```python
from build123d import *

# Parameters (mm, degrees)
F1_DEPTH = 0.635


# Not quite as in the source:
# - a feature names something its author has since deleted; it is built from what else it names


with BuildPart() as f1:
    # F0 (on Top) → F1 (new body)
    with BuildSketch(Plane.XY):
        with BuildLine():
            ThreePointArc((107.95, 0), (107.0200640303, 2.2450640303), (104.775, 3.175))
            Line((104.775, 3.175), (-69.215, 3.175))
            Line((-69.215, 3.175), (-74.295, 3.175))
            Line((-74.295, 3.175), (-74.295, -3.175))
            Line((-74.295, -3.175), (-69.215, -3.175))
            Line((-69.215, -3.175), (104.775, -3.175))
            ThreePointArc((104.775, -3.175), (107.0200640303, -2.2450640303), (107.95, 0))
        make_face()
        with BuildLine():
            Line((-74.295, -3.175), (-74.295, 3.175))
            Line((-74.295, 3.175), (-79.375, 3.175))
            Line((-79.375, 3.175), (-104.775, 3.175))
            ThreePointArc((-104.775, 3.175), (-107.0200640303, 2.2450640303), (-107.95, 0))
            ThreePointArc((-107.95, 0), (-107.0200640303, -2.2450640303), (-104.775, -3.175))
            Line((-104.775, -3.175), (-79.375, -3.175))
            Line((-79.375, -3.175), (-74.295, -3.175))
        make_face()
        with BuildLine():
            Line((-74.295, 9.525), (-69.215, 9.525))
            Line((-69.215, 9.525), (104.775, 9.525))
            ThreePointArc((104.775, 9.525), (107.0200640303, 10.4549359697), (107.95, 12.7))
            ThreePointArc((107.95, 12.7), (107.0200640302, 14.9450640302), (104.775, 15.875))
            Line((104.775, 15.875), (-74.295, 15.875))
            Line((-74.295, 15.875), (-74.295, 9.525))
        make_face()
        with BuildLine():
            Line((-79.375, 9.525), (-74.295, 9.525))
            Line((-74.295, 9.525), (-74.295, 15.875))
            Line((-74.295, 15.875), (-104.775, 15.875))
            ThreePointArc((-104.775, 15.875), (-107.0200640302, 14.9450640302), (-107.95, 12.7))
            ThreePointArc((-107.95, 12.7), (-107.0200640303, 10.4549359697), (-104.775, 9.525))
            Line((-104.775, 9.525), (-79.375, 9.525))
        make_face()
        with BuildLine():
            Line((-69.2150000001, -9.5250000001), (-74.295, -9.5250000001))
            Line((-74.295, -9.5250000001), (-74.295, -15.875))
            Line((-74.295, -15.875), (104.775, -15.875))
            ThreePointArc((104.775, -15.875), (107.0200640302, -14.9450640302), (107.95, -12.7))
            ThreePointArc((107.95, -12.7), (107.0200640303, -10.4549359697), (104.775, -9.525))
            Line((104.775, -9.5250000001), (-69.2150000001, -9.5250000001))
        make_face()
        with BuildLine():
            Line((-74.295, -15.875), (-74.295, -9.5250000001))
            Line((-74.295, -9.5250000001), (-79.375, -9.5250000001))
            Line((-79.375, -9.5250000001), (-104.775, -9.5250000001))
            ThreePointArc((-104.775, -9.525), (-107.0200640303, -10.4549359697), (-107.95, -12.7))
            ThreePointArc((-107.95, -12.7), (-107.0200640302, -14.9450640302), (-104.775, -15.875))
            Line((-104.775, -15.875), (-74.295, -15.875))
        make_face()
        with BuildLine():
            Line((-79.375, 3.175), (-74.295, 3.175))
            Line((-74.295, 3.175), (-74.295, 9.525))
            Line((-74.295, 9.525), (-79.375, 9.525))
            ThreePointArc((-79.375, 9.525), (-77.98351653, 6.35), (-79.375, 3.175))
        make_face()
        with BuildLine():
            Line((-74.295, 3.175), (-69.215, 3.175))
            ThreePointArc((-69.215, 3.175), (-70.6064834701, 6.35), (-69.215, 9.525))
            Line((-69.215, 9.525), (-74.295, 9.525))
            Line((-74.295, 9.525), (-74.295, 3.175))
        make_face()
        with BuildLine():
            Line((-74.295, -9.5250000001), (-74.295, -3.175))
            Line((-74.295, -3.175), (-79.375, -3.175))
            ThreePointArc((-79.375, -3.175), (-77.9835165299, -6.35), (-79.375, -9.525))
            Line((-79.375, -9.5250000001), (-74.295, -9.5250000001))
        make_face()
        with BuildLine():
            Line((-69.215, -3.175), (-74.295, -3.175))
            Line((-74.295, -3.175), (-74.295, -9.5250000001))
            Line((-74.295, -9.5250000001), (-69.2150000001, -9.5250000001))
            ThreePointArc((-69.2150000001, -9.525), (-70.6064834702, -6.35), (-69.215, -3.175))
        make_face()
    extrude(amount=F1_DEPTH)


solid = f1.part
```
The listing builds one solid part. Answer for the finished solid, in the listing's coordinates (mm). Give positions to 0.01 mm unless a question says otherwise; leave off trailing zeros. Order: outer loops, then holes, each group sorted by start corner. A loop starts at its lowest first (then second) coordinate and runs counter-clockwise, first axis right, second up. Notation, with made-up numbers: (-26.75, -12) -> (13.25, -12) arc R32 cw to (13.25, 17) -> close; hole circle Ø2 at (49.25, 8.5). An arc over 180 degrees is marked (long way). One line per item, written item: value.
1) Find section A-A, the plane x = -15. Determine the outline of the cut face in (y, z) (3 decimals), plus the area to 3 significant figures.
Reported:
outline: (-15.875, 0) -> (-9.525, 0) -> (-9.525, 0.635) -> (-15.875, 0.635) -> close; (-3.175, 0) -> (3.175, 0) -> (3.175, 0.635) -> (-3.175, 0.635) -> close; (9.525, 0) -> (15.875, 0) -> (15.875, 0.635) -> (9.525, 0.635) -> close
area: 12.1 mm^2
2) Find the intervals of material crossed by line 1 (Y direction, x = 47, z = 0.45) (3 decimals); line 2 (X direction, y = -6, z = 0.25); line 3 (X direction, y = -13, z = 0.15), in increasing order.
Reported:
line 1: y = -15.875 to -9.525, -3.175 to 3.175, 9.525 to 15.875
line 2: x = -78 to -70.59
line 3: x = -107.94 to 107.94
3) Find section C-C, the plane y = 6. Determine the outline of the cut face in (x, z) (3 decimals), plus the area to 3 significant figures.
Reported:
outline: (-77.998, 0) -> (-70.592, 0) -> (-70.592, 0.635) -> (-77.998, 0.635) -> close
area: 4.70 mm^2
4) Find section B-B, the plane z = 0.4. Determine the outline of the cut face in (x, y) (3 decimals).
Reported:
outline: (-104.775, -15.875) -> (104.775, -15.875) arc R3.175 ccw to (104.775, -9.525) -> (-69.215, -9.525) arc R4.318 cw to (-69.215, -3.175) -> (104.775, -3.175) arc R3.175 ccw to (104.775, 3.175) -> (-69.215, 3.175) arc R4.318 cw to (-69.215, 9.525) -> (104.775, 9.525) arc R3.175 ccw to (104.775, 15.875) -> (-104.775, 15.875) arc R3.175 ccw to (-104.775, 9.525) -> (-79.375, 9.525) arc R4.318 cw to (-79.375, 3.175) -> (-104.775, 3.175) arc R3.175 ccw to (-104.775, -3.175) -> (-79.375, -3.175) arc R4.318 cw to (-79.375, -9.525) -> (-104.775, -9.525) arc R3.175 ccw to start
5) A flat-ended cylindrical pin translates along its axis: P1, Ø10, axis at x = -56.5, y = 3, coming from the -Z side. Find the tip coordinate at first contact, or state that the pin passes through.
Reported:
P1: stops at z = 0
6) Find section D-D, the plane y = -7.5. Determine the outline of the cut face in (x, z) (3 decimals), plus the area to 3 significant figures.
Reported:
outline: (-78.139, 0) -> (-70.451, 0) -> (-70.451, 0.635) -> (-78.139, 0.635) -> close
area: 4.88 mm^2
